Part model, mm, in its own coordinate system. A direction names the side the tool comes from. Coordinates: 2 decimals unless noted, no trailing zeros. Write each loop counter-clockwise with the first axis right and the second up, starting at its lowest first coordinate (ties: lowest second). Pieces come first, ordered by that corner, then holes. Notation, with made-up numbers: (0.25, 3.5) -> (15.25, 3.5) arc R7 ccw to (15.25, 11.5) -> close; hole circle Ø2 at (64, 26). An arc over 180 degrees is marked (long way). Write item = value, one per line.
Autodesk Inventor part; units mm, degrees
ref_plane "YZ Plane" through (0, 0, 0) normal (1, 0, 0) x (0, 1, 0)
ref_plane "XZ Plane" through (0, 0, 0) normal (0, 1, 0) x (-1, 0, 0)
ref_plane "XY Plane" through (0, 0, 0) normal (0, 0, 1) x (1, 0, 0)
sketch "Skizze1" plane through (0, 0, 0) normal (0, 0, 1) x (1, 0, 0)
  line L0 (0, 15.4) -> (0, -15.4) construction
  line L1 (-15.4, 0) -> (15.4, 0) construction
  circle A0 centre (0, 0) radius 1.9
  arc A1 (-4.4, -4.1564) -> (4.4, -4.1564) centre (0, -2) ccw
  line L2 (0, 2) -> (0, 0) construction
  line L3 (0, 0) -> (2, 0) construction
  arc A2 (-4.4, -0.1564) -> (4.4, -0.1564) centre (0, 2) ccw
  arc A3 (4.4, 0.1564) -> (-4.4, 0.1564) centre (0, -2) ccw
  line L4 (0, 0) -> (0, -2) construction
  circle A4 centre (0, 0) radius 9.5
  circle A5 centre (0, 0) radius 11
  circle A6 centre (0, 0) radius 6.35 construction
  circle A7 centre (0, -6.35) radius 1.5
  circle A8 centre (0, 6.35) radius 1.5
  line L5 (0, -6.35) -> (0, 0) construction
  line L6 (0, 0) -> (-6.35, 0) construction
  line L7 (4.4, 4.1564) -> (4.4, -4.1564)
  line L8 (-4.4, 4.1564) -> (-4.4, -4.1564)
  line L9 (4.9, 2) -> (4.9, -2) construction
  arc A9 (4.4, 4.1564) -> (-4.4, 4.1564) centre (0, 2) ccw
  arc A10 (4.4, -0.1564) -> (4.4, 4.1564) centre (0, 2) ccw construction
  arc A11 (4.4, -4.1564) -> (4.4, 0.1564) centre (0, -2) ccw construction
  arc A12 (-4.4, 4.1564) -> (-4.4, -0.1564) centre (0, 2) ccw construction
  arc A13 (-4.4, 0.1564) -> (-4.4, -4.1564) centre (0, -2) ccw construction
  line L10 (-4.9, 2) -> (-4.9, -2) construction
  circle A14 centre (0, 0) radius 2.4
  circle A15 centre (0, 2) radius 5.9
  circle A16 centre (0, -6.35) radius 2.5
  circle A17 centre (0, 6.35) radius 2.5
  circle A18 centre (0, -2) radius 5.9
  circle A19 centre (0, 0) radius 4.9
  dimension "d0" = 3.8
  dimension "d1" = 2
  dimension "d14" = 2
  dimension "d15" = 180
  dimension "d16" = 9.5
  dimension "d17" = 1.5
  dimension "d20" = 6.35
  dimension "d21" = 3
  dimension "d26" = 0.5
  dimension "d27" = 0.5
  dimension "d28" = 4.9
  dimension "d31" = 0.5
  dimension "d34" = 1
  dimension "d37" = 1
  dimension "d40" = 1
extrude "Extrusion6" add sketch "Skizze1" along normal blind 3 contours A5
extrude "Extrusion7" add sketch "Skizze1" along normal blind 1.5 from surface at 3 contours A0 | L8 A19 A16 A1 | A1 A16 A18 A15 A19 L8 | A16 A19 A7 A1 | A1 A7 A16 A18 | A19 A15 L8 | L8 A15 A16 A19 | A7 A19 A1 | A1 A7 | A16 A15 A19 A7 | A18 A16 | A15 A19 A18 L8 | L8 A2 L7 A15 A16 | A15 A18 A19 | A7 A19 A16 A1 | A7 A19 | A16 A15 | A16 A1 L7 A19 A15 A18 | A15 A17 A9 L8 A19 A18 | L8 A3 L7 A2 | A19 L8 A18 | A16 A19 L7 A1 | A15 L7 A19 A16 | A17 A15 | A15 A17 A9 A8 | L7 A18 A19 A15 | L8 A18 A17 L7 A3 | L8 A19 A17 A18 | L8 A9 A17 A19 | A15 A19 L7 | A18 A19 L7 A9 A17 A15 | A15 A19 A18 | A9 A8 A19 A17 | A18 A17 | A17 A19 A8 A18 | A18 L7 A19 | A9 A8 A19 | A8 A9 | A18 A17 A19 L7 | A19 A8 | A19 A17 A9 L7 | A17 A19 A8 A9 | A4 | A5 | A14
extrude "Extrusion15" add sketch "Skizze1" along normal blind 4 from surface at 4.5 contours A0 | A19 A15 L8 | L8 A15 A16 A19 | A16 A15 A19 A7 | A15 A19 A18 L8 | L8 A2 L7 A15 A16 | A7 A19 | A16 A15 | L8 A3 L7 A2 | A19 L8 A18 | A15 L7 A19 A16 | L7 A18 A19 A15 | L8 A18 A17 L7 A3 | L8 A19 A17 A18 | A15 A19 L7 | A18 A17 | A17 A19 A8 A18 | A18 L7 A19 | A18 A17 A19 L7 | A19 A8 | A14
extrude "Extrusion8" cut sketch "Skizze1" along normal through all both and the other way through all contours A7 A19 A1 | A1 A7 | A7 A19 | A9 A8 A19 | A8 A9 | A19 A8
extrude "Extrusion16" add sketch "Skizze1" along normal blind 4 from surface at 8.5 contours A0 | L8 A3 L7 A2 | A14
extrude "Extrusion12" cut sketch "Skizze1" along normal blind 3 from surface at 12.5 contours A16 A19 A7 A1 | A1 A7 A16 A18 | A16 A15 A19 A7 | A18 A16 | A7 A19 A16 A1 | A16 A15 | A17 A15 | A15 A17 A9 A8 | A9 A8 A19 A17 | A18 A17 | A17 A19 A8 A18 | A9 A8 A19 | A8 A9 | A19 A8 | A17 A19 A8 A9
extrude "Extrusion2" add sketch "Skizze1" along normal blind 4 from surface at 12.5 contours A0 | L8 A3 L7 A2 | L8 A18 A17 L7 A3 | L8 A19 A17 A18 | L8 A9 A17 A19 | A9 A8 A19 A17 | A18 A17 | A17 A19 A8 A18 | A9 A8 A19 | A18 A17 A19 L7 | A19 A8 | A19 A17 A9 L7 | A17 A19 A8 A9 | A14
extrude "Extrusion3" add sketch "Skizze1" along normal blind 3 from surface at 16.5 contours A0 | L8 A3 L7 A2 | A14
extrude "Extrusion4" add sketch "Skizze1" along normal blind 4 from surface at 19.5 contours A0 | L8 A19 A16 A1 | A16 A19 A7 A1 | L8 A15 A16 A19 | A7 A19 A1 | A16 A15 A19 A7 | L8 A2 L7 A15 A16 | A7 A19 A16 A1 | A7 A19 | A16 A15 | L8 A3 L7 A2 | A16 A19 L7 A1 | A15 L7 A19 A16 | A14
extrude "Extrusion10" add sketch "Skizze1" along normal blind 1 from surface at 23.5 contours A0 | A14
extrude "Extrusion14" add sketch "Skizze1" along normal blind 10 from surface at 24.5 contours A0
equation "\"d14\" = d1"
equation "\"d27\" = d26"
properties part number "ExcentricShaft"
Q1. Probe line 1 (Z direction, x = -2.75, y = 4.75); line 2 (Y direction, x = 0, z = 1.2); line 3 (Z direction, x = -9.25, y = -4). List the from-to ranges inside material, lowest first. Write a range as from..to.
Model answer:
line_1 = 3..4.5, 12.5..16.5
line_2 = -11..-9.5, 9.5..11
line_3 = 0..4.5
Q2. Saw through at D-D on y = 9. Give the cut face in (x, z), and give its area (3 significant figures).
Model answer:
outline = (-6.32, 0) -> (-3.04, 0) -> (-3.04, 3) -> (3.04, 3) -> (3.04, 0) -> (6.32, 0) -> (6.32, 4.5) -> (-6.32, 4.5) -> close
area = 38.7 mm²
Q3. Saw through at C-C on x = -5.75. Give the cut face in (y, z).
Model answer:
outline = (-9.38, 0) -> (-7.56, 0) -> (-7.56, 3) -> (7.56, 3) -> (7.56, 0) -> (9.38, 0) -> (9.38, 4.5) -> (-9.38, 4.5) -> close
Q4. Pin check, flat tips, straight feed: pin 1 (2 mm diameter, centred on x = -1, y = 4, fed in from +Z); pin 2 (2.5 mm diameter, centred on x = 0, y = 6.35, fed in from -Z); pin 3 (8 mm diameter, centred on x = 1, z = 9.5, fed in from -Y). Stop position of each tip, or through.
Model answer:
pin_1 = 16.5
pin_2 = 12.5
pin_3 = -4.89
Q5. Mould opens along X. For faces 5 (the face through (4.4, 0, 18)), 6 (the face through (0, 0, 3)), 7 (the face through (-0.1, 6.9, 14.5)), 8 (the face through (-0.195, 4.863, 3.878)) say: released by +X, released by -X, zero draft, split by the parting line, or undercut.
Model answer:
face_5 = released by +X
face_6 = undercut
face_7 = split by the parting line
face_8 = undercut
Q6. Saw through at A-A on y = 6.35. Give the cut face in (x, z), and give its area (3 significant figures).
Model answer:
outline = (-8.98, 0) -> (-7.07, 0) -> (-7.07, 3) -> (-1.5, 3) -> (-1.5, 4.5) -> (-8.98, 4.5) -> close; (-2.26, 12.5) -> (2.26, 12.5) -> (2.26, 16.5) -> (-2.26, 16.5) -> close; (1.5, 3) -> (7.07, 3) -> (7.07, 0) -> (8.98, 0) -> (8.98, 4.5) -> (1.5, 4.5) -> close
area = 52.0 mm²
Q7. Saw through at B-B on z = 17.5. Give the cut face in (x, y), and give its area (3 significant figures).
Model answer:
outline = (-4.4, -0.16) arc R4.9 ccw to (4.4, -0.16) -> (4.4, 0.16) arc R4.9 ccw to (-4.4, 0.16) -> close
area = 37.3 mm²
Q8. Which spindle directions (+Z, -Z, +X, -X, +Y, -Y) get a long thin tool onto all of the face, cutting with end or side? Do faces 1 (the face through (0, 4, 12.5)), 2 (the face through (-4.9, -0.1, 6.5)), 3 (the face through (-0.1, -3.2, 8.5)), 4 (the face through (4.38, 8.43, 1.48)). Say none if no direction does.
Model answer:
face_1 = +Y
face_2 = -X
face_3 = none
face_4 = -Z
